```python
from build123d import *

# Parameters (mm, degrees)
SKETCH_3_W          = 12.1
SKETCH_3_H          = 5.5
EXTRUDE_1_DEPTH     = 6
SKETCH_4_W          = 6.24
SKETCH_4_H          = 3.15
CUT_EXTRUDE_1_DEPTH = 1
SKETCH_5_W          = 3
SKETCH_5_H          = 3
EXTRUDE_2_DEPTH     = 6
CUT_EXTRUDE_2_REACH = 18.896
SKETCH_7_W          = 1
SKETCH_7_H          = 0.46
SKETCH_7_W_2        = 0.45
SKETCH_7_H_2        = 1.5
EXTRUDE_3_DEPTH     = 3
FILLET_1_R          = 0.3


with BuildPart() as part:
    # Sketch 3 → Extrude 1 (new body)
    with BuildSketch(Plane.XY):
        with Locations((6.05, 2.75)):
            Rectangle(SKETCH_3_W, SKETCH_3_H)
    extrude(amount=EXTRUDE_1_DEPTH)

    # Sketch 4 → Cut-Extrude 1 (cut)
    with BuildSketch(Plane.XY.offset(6)):
        with Locations((6.05, 2.75)):
            Rectangle(SKETCH_4_W, SKETCH_4_H)
    extrude(amount=-CUT_EXTRUDE_1_DEPTH, mode=Mode.SUBTRACT)

    # Sketch 5 → Extrude 2 (add)
    with BuildSketch(Plane.XY.offset(5)):
        with Locations((4.53, 2.75)):
            Rectangle(SKETCH_5_W, SKETCH_5_H)
    extrude(amount=EXTRUDE_2_DEPTH)

    # Sketch 6 → Cut-Extrude 2 (cut, up to next)
    with BuildSketch(Plane.XZ.offset(-1.25), mode=Mode.PRIVATE) as cut_extrude_2_sk1:
        Polygon((3.03, 11), (3.33, 10.7), (3.63, 11), align=None)
    cut_extrude_2_tool1 = extrude(cut_extrude_2_sk1.sketch, amount=-CUT_EXTRUDE_2_REACH, mode=Mode.PRIVATE) & part.part
    # Sketch 6 → Cut-Extrude 2 (cut, up to next)
    with BuildSketch(Plane.XZ.offset(-1.25), mode=Mode.PRIVATE) as cut_extrude_2_sk2:
        Polygon((4.13, 10.7), (4.43, 11), (3.83, 11), align=None)
    cut_extrude_2_tool2 = extrude(cut_extrude_2_sk2.sketch, amount=-CUT_EXTRUDE_2_REACH, mode=Mode.PRIVATE) & part.part
    # Sketch 6 → Cut-Extrude 2 (cut, up to next)
    with BuildSketch(Plane.XZ.offset(-1.25), mode=Mode.PRIVATE) as cut_extrude_2_sk3:
        Polygon((4.93, 10.7), (5.23, 11), (4.63, 11), align=None)
    cut_extrude_2_tool3 = extrude(cut_extrude_2_sk3.sketch, amount=-CUT_EXTRUDE_2_REACH, mode=Mode.PRIVATE) & part.part
    # Sketch 6 → Cut-Extrude 2 (cut, up to next)
    with BuildSketch(Plane.XZ.offset(-1.25), mode=Mode.PRIVATE) as cut_extrude_2_sk4:
        Polygon((5.73, 10.7), (6.03, 11), (5.43, 11), align=None)
    cut_extrude_2_tool4 = extrude(cut_extrude_2_sk4.sketch, amount=-CUT_EXTRUDE_2_REACH, mode=Mode.PRIVATE) & part.part
    add(cut_extrude_2_tool1.solids().sort_by_distance((3.33, 1.25, 10.9))[0], mode=Mode.SUBTRACT)
    add(cut_extrude_2_tool2.solids().sort_by_distance((4.13, 1.25, 10.9))[0], mode=Mode.SUBTRACT)
    add(cut_extrude_2_tool3.solids().sort_by_distance((4.93, 1.25, 10.9))[0], mode=Mode.SUBTRACT)
    add(cut_extrude_2_tool4.solids().sort_by_distance((5.73, 1.25, 10.9))[0], mode=Mode.SUBTRACT)

    # Sketch 7 → Extrude 3 (add)
    with BuildSketch(Plane(origin=(0, 0, 0), x_dir=(-1, 0, 0), z_dir=(0, 0, -1))):
        with Locations((-3.05, 2.75)):
            Rectangle(SKETCH_7_W, SKETCH_7_H)
        with Locations((-6.05, 2.75)):
            Rectangle(SKETCH_7_W, SKETCH_7_H)
        with Locations((-9.05, 2.75)):
            Rectangle(SKETCH_7_W, SKETCH_7_H)
        with Locations((-11.875, 2.75)):
            Rectangle(SKETCH_7_W_2, SKETCH_7_H_2)
        with Locations((-0.225, 2.75)):
            Rectangle(SKETCH_7_W_2, SKETCH_7_H_2)
    extrude(amount=EXTRUDE_3_DEPTH)

    # Fillet 1
    fillet_1_edges = [part.edges().sort_by_distance(p)[0] for p in [
        (12.1, 2.75, 6),
        (6.05, 5.5, 6),
        (0, 2.75, 6),
        (6.05, 0, 6),
        (0, 5.5, 3),
        (12.1, 5.5, 3),
        (12.1, 0, 3),
        (0, 0, 3),
    ]]
    fillet(fillet_1_edges, radius=FILLET_1_R)


solid = part.part
```
Check sheet for the modelled part. Datum: model origin and axes. Units: mm. A direction names the side the tool comes from. Round coordinates to 2 decimals unless told otherwise and drop trailing zeros. Order: outer loops, then holes, each group sorted by start corner. A loop starts at its lowest first (then second) coordinate and runs counter-clockwise, first axis right, second up.
1) Mould release check, pull along X, two halves, no side actions. Record for faces 1 (the flat face through (6, 2.98, -1)), 2 (the flat face through (6, 5.5, 3)), 3 (the flat face through (0, 3, 2)): +X half, -X half, draft (parallel to the pull), parting line (faces both ways), or undercut.
2) Section check B-B (x = 7.5). Record the boundary of the cut face in (y, z) (3 decimals).
3) Section check D-D (x = 1.75). Record the boundary of the cut face in (y, z).
4) Scan lines: line 1 (Z direction, x = 3.75, y = 3); line 2 (Z direction, x = 3, y = 0.4); line 3 (X direction, y = 5.25, z = 2.5). Record each from-to range of solid material in increasing order.
5) Section check A-A (y = 4.65). Record the boundary of the cut face in (x, z).
6) Section check C-C (z = 7). Record the boundary of the cut face in (x, y), and give its area (3 significant figures).
7) Tool access check on faces 4 (the flat face through (12.1, 3, 2)), 5 (the flat face through (9.17, 2.7, 5.5)), 6 (the flat face through (0.45, 3, -1)), 7 (the flat face through (6, 0, 3)), 8 (the flat face through (9, 2.52, -1)). Record the directions out of +Z, -Z, +X, -X, +Y, -Y that give a thin tool (end or side, any length) a straight path to the whole face; none if there is none.
8) Go/stop test with flat-tipped pins: pin 1 Ø2 at (x, y) = (2, 4) entering from -Z; pin 2 Ø1 at (y, z) = (1.5, 7.5) entering from -X; pin 3 Ø0.5 at (x, z) = (3, -1) entering from -Y. Record where each tip stops, or that it passes through.
Result:
1. face 1: undercut
1. face 2: draft
1. face 3: -X half
2. outline: (0, 0) - (5.5, 0) - (5.5, 5.7) arc R0.3 ccw to (5.2, 6) - (4.325, 6) - (4.325, 5) - (1.175, 5) - (1.175, 6) - (0.3, 6) arc R0.3 ccw to (0, 5.7) - close
3. outline: (0, 0) - (5.5, 0) - (5.5, 5.7) arc R0.3 ccw to (5.2, 6) - (0.3, 6) arc R0.3 ccw to (0, 5.7) - close
4. line 1: z = 0 to 11
4. line 2: z = 0 to 6
4. line 3: x = 0 to 12.1
5. outline: (0, 0) - (12.1, 0) - (12.1, 5.7) arc R0.3 ccw to (11.8, 6) - (0.3, 6) arc R0.3 ccw to (0, 5.7) - close
6. outline: (3.03, 1.25) - (6.03, 1.25) - (6.03, 4.25) - (3.03, 4.25) - close
6. area: 9.00 mm2
7. face 4: +Z, -Z, +X, +Y, -Y
7. face 5: +Z
7. face 6: -Z, +Y, -Y
7. face 7: +Z, -Z, +X, -X, -Y
7. face 8: -Z, -Y
8. pin 1: stops at z = 0
8. pin 2: stops at x = 3.03
8. pin 3: stops at y = 2.52
